Study the drawing (mm; zero at the part's minimum x, y, z) and answer. A direction names the side the tool comes from. Coordinates: 2 decimals unless noted, no trailing zeros. Loops run counter-clockwise (first coordinate to the right, second up) from the corner with the lowest first, then second, coordinate; pieces in that order, holes last. Notation, with made-up numbers: (17.5, 45) - (31.5, 45) arc R26 ccw to (31.5, 63) - close; hole circle Ø2 at (85.5, 76). An arc over 180 degrees is marked (long way). Use one line per item in the form item = value.
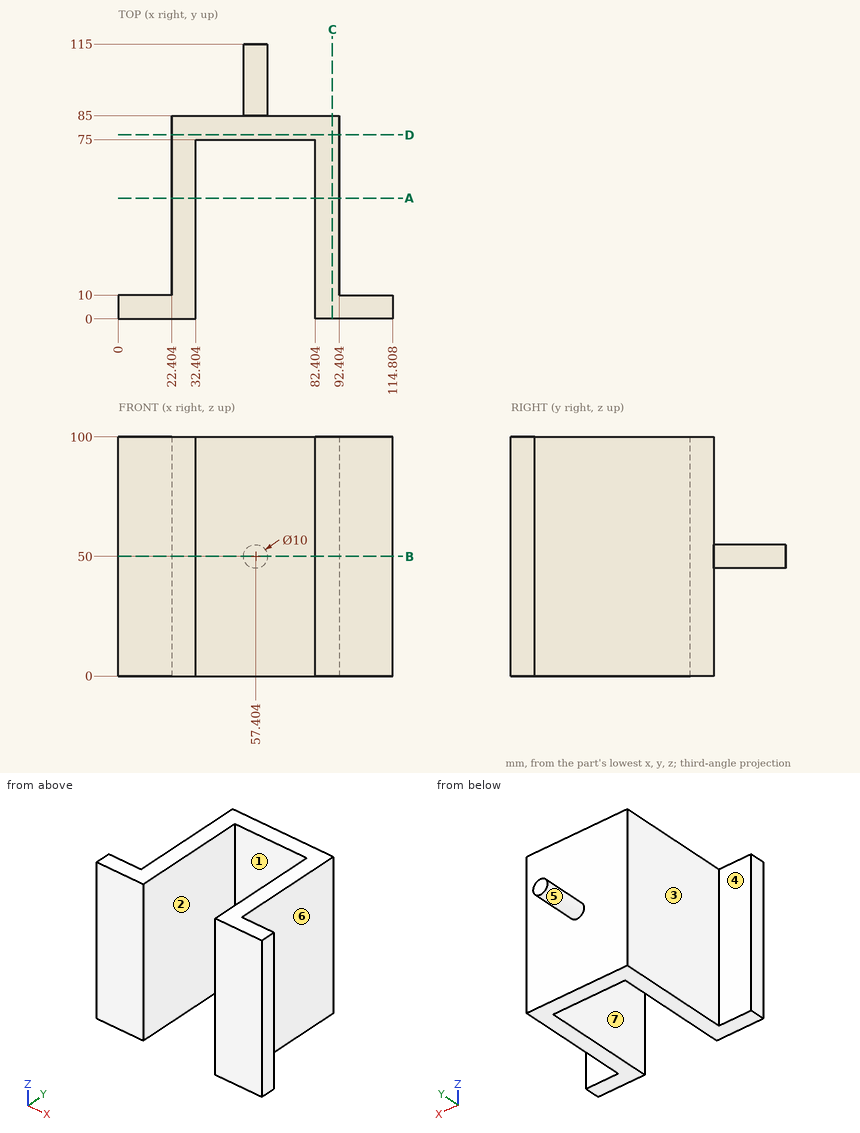
Item 1: Which of the six approach directions +Z, -Z, +X, -X, +Y, -Y give full straight-line access (tool end or side, diameter ignored) to the marked faces 5, 6 and 7?
Results below:
face_5 = +Y
face_6 = +Z, -Z, +X, +Y
face_7 = +Z, -Z, -Y
Item 2: The part is cut by section B-B on z = 50. Give the vertices of the cut face in (x, y).
Results below:
outline = (0, 0) - (32.4, 0) - (32.4, 75) - (82.4, 75) - (82.4, 0) - (114.81, 0) - (114.81, 10) - (92.4, 10) - (92.4, 85) - (62.4, 85) - (62.4, 115) - (52.4, 115) - (52.4, 85) - (22.4, 85) - (22.4, 10) - (0, 10) - close
Item 3: The part is cut by section A-A on y = 50.5. Give the vertices of the cut face in (x, z), plus the area to 3 significant figures.
Results below:
outline = (22.4, 0) - (32.4, 0) - (32.4, 100) - (22.4, 100) - close; (82.4, 0) - (92.4, 0) - (92.4, 100) - (82.4, 100) - close
area = 2,000 mm²
Item 4: The part is cut by section C-C on x = 89.5. Give the vertices of the cut face in (y, z), plus the area to 3 significant figures.
Results below:
outline = (0, 0) - (85, 0) - (85, 100) - (0, 100) - close
area = 8,500 mm²
Item 5: Find the intervals of material crossed by L1, parallel to X at y = 43, z = 40; L2, parallel to X at y = 80, z = 58.5; L3, parallel to Y at x = 106, z = 83, in increasing order.
Results below:
L1 = 22.4 to 32.4, 82.4 to 92.4
L2 = 22.4 to 92.4
L3 = 0 to 10
Item 6: Each of these flat-tipped pins is pushed along its axis until it touches: P1, Ø11, axis at x = 15, z = 38.5, coming from the +Y side; P2, Ø1.5, axis at x = 64, z = 21, coming from the +Y side; P3, Ø5, axis at x = 58, z = 57, coming from the +Y side; P4, Ø4, axis at x = 46, z = 47, coming from the -Y side. Where does it stop, or does it pass through?
Results below:
P1 = 10
P2 = 85
P3 = 115
P4 = 75
Item 7: For a pull along X with two mould halves and no side action, classify the marked faces 1, 2, 3 and 4 as +X half, -X half, draft (parallel to the pull), parting line (faces both ways), or undercut.
Results below:
face_1 = undercut
face_2 = undercut
face_3 = -X half
face_4 = draft
Item 8: The part is cut by section D-D on y = 77. Give the vertices of the cut face in (x, z), plus the area to 3 significant figures.
Results below:
outline = (22.4, 0) - (92.4, 0) - (92.4, 100) - (22.4, 100) - close
area = 7,000 mm²
